Geometry: final body of the model. Coordinates: model frame, mm. A direction names the side the tool comes from. Give positions to 0.01 mm unless a question says otherwise; leave off trailing zeros. Order: outer loops, then holes, each group sorted by start corner. A loop starts at its lowest first (then second) coordinate and runs counter-clockwise, first axis right, second up. Notation, with made-up numbers: (23.5, 19) - (62.5, 19) arc R21 cw to (62.5, 29) - close; hole circle Ø3 at (-20, 60). An arc over 180 degrees is marked (long way). Put each result on its own line as item: value. Start each with the question number.
1. Section C-C on z = 15. Return the cut outline in (x, y).
2. Set-up query: faces 1 (the flat face through (-18, 5, 17)), 2 (the cylindrical face through (-13.38, 11.51, 2.53)). Return all of +Z, -Z, +X, -X, +Y, -Y with unobstructed straight access to the full face (end or side cutting, diameter ignored); none if empty.
3. First-contact query: P1, Ø6, axis at x = -15, z = 15, coming from the +Y side; P2, Ø6, axis at y = 11.5, z = 15.5, coming from the -X side; P3, Ø12.5, axis at x = -13, y = 15.5, coming from the +Z side. Flat tips, straight axial feed; report the tip coordinate or a pass-through.
4. Section B-B on x = -15. Return the cut outline in (y, z), plus the area to 4 significant figures.
5. Section A-A on y = 15. Return the cut outline in (x, z).
6. Mould query, pull axis X, two halves, no side actions, for faces 3 (the cylindrical face through (-15.86, 2.47, 12.92)), 4 (the flat face through (-30, 8.1, 4.8)), 5 (the cylindrical face through (-2.465, 16.996, 16.038)). Classes: pulls with the +X half, pulls with the -X half, needs draft (parallel to the pull), parting line crosses it, or undercut.
7. Section D-D on x = -2. Return the cut outline in (y, z), plus the area to 3 significant figures.
8. Ray query, line 1 along Z through (x, y) = (-2.75, 15); line 2 along X through (y, z) = (3.25, 15). Return the intervals inside material, ascending. Write a range as from..to.
from build123d import *

# Parameters (mm, degrees)
ESBO_O1_W                         = 30
ESBO_O1_H                         = 30
RESSALTO_EXTRUS_O1_DEPTH          = 30
ESBO_O3_W                         = 25
ESBO_O3_H                         = 25
CORTE_EXTRUS_O2_DEPTH             = 25
FURO_COM_FOLGA_DE_M41_D           = 4.5
FURO_COM_FOLGA_DE_M41_ON_FACE_2_D = 4.5
FURO_COM_FOLGA_DE_M32_D           = 3.4


with BuildPart() as part:
    # Esboço1 → Ressalto-extrusão1 (new body)
    with BuildSketch(Plane.XY):
        with Locations((-15, 15)):
            Rectangle(ESBO_O1_W, ESBO_O1_H)
    extrude(amount=RESSALTO_EXTRUS_O1_DEPTH)

    # Esboço3 → Corte-extrusão2 (cut)
    with BuildSketch(Plane(origin=(0, 30, 0), x_dir=(1, 0, 0), z_dir=(0, 1, 0))):
        with Locations((-17.5, -17.5)):
            Rectangle(ESBO_O3_W, ESBO_O3_H)
    extrude(amount=-CORTE_EXTRUS_O2_DEPTH, mode=Mode.SUBTRACT)

    # Furo com folga de M41 (through all)
    with Locations(Plane(origin=(-5, 15, 15), x_dir=(0, 0, -1), z_dir=(-1, 0, 0))):
        with Locations((0, 0)):
            Hole(FURO_COM_FOLGA_DE_M41_D / 2)

    # Furo com folga de M41 on face 2 (through all)
    with Locations(Plane(origin=(-15, 5, 15), x_dir=(0, 0, 1), z_dir=(0, 1, 0))):
        with Locations((0, 0)):
            Hole(FURO_COM_FOLGA_DE_M41_ON_FACE_2_D / 2)

    # Furo com folga de M32 (through all)
    with Locations(Plane(origin=(-15.001293069, 10.996070653, 0), x_dir=(-1, 0, 0), z_dir=(0, 0, -1))):
        with Locations((0, 0)):
            Hole(FURO_COM_FOLGA_DE_M32_D / 2)


solid = part.part
Resolved:
1. outline: (-30, 0) - (-17.25, 0) - (-17.25, 5) - (-30, 5) - close; (-12.75, 0) - (0, 0) - (0, 12.75) - (-5, 12.75) - (-5, 5) - (-12.75, 5) - close; (-5, 17.25) - (0, 17.25) - (0, 30) - (-5, 30) - close
2. face 1: +Z, -X, +Y
2. face 2: +Z, -Z
3. P1: y = 5
3. P2: x = -5
3. P3: z = 5
4. outline: (0, 0) - (9.3, 0) - (9.3, 5) - (5, 5) - (5, 12.75) - (0, 12.75) - close; (0, 17.25) - (5, 17.25) - (5, 30) - (0, 30) - close; (12.7, 0) - (30, 0) - (30, 5) - (12.7, 5) - close
4. area: 235.5 mm^2
5. outline: (-30, 0) - (0, 0) - (0, 12.75) - (-5, 12.75) - (-5, 5) - (-30, 5) - close; (-5, 17.25) - (0, 17.25) - (0, 30) - (-5, 30) - close
6. face 3: undercut
6. face 4: pulls with the -X half
6. face 5: needs draft
7. outline: (0, 0) - (30, 0) - (30, 30) - (0, 30) - close; hole circle Ø4.5 at (15, 15)
7. area: 884 mm^2
8. line 1: 0..12.75, 17.25..30
8. line 2: -30..-17.25, -12.75..0
